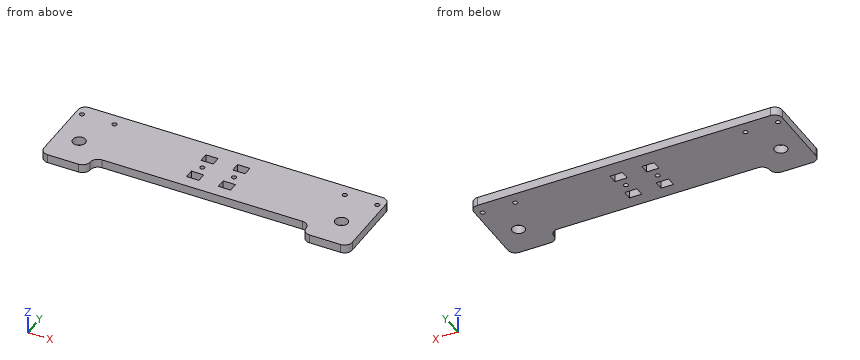
```python
from build123d import *

# Parameters (mm, degrees)
F0_W     = 200
F0_H     = 52
F0_R     = 4.1
F0_W_2   = 8
F0_H_2   = 6
F0_R_2   = 1.5
F1_DEPTH = 5.588
F2_W     = 140
F2_H     = 10
F3_DEPTH = 25
F4_R     = 4.99999


# Not quite as in the source:
# - a fillet or chamfer is up to 0.001 mm smaller than in the source, because OpenCascade refuses the exact size


with BuildPart() as f1:
    # F0 (on Top) → F1 (new body)
    with BuildSketch(Plane.XY):
        Rectangle(F0_W, F0_H)
        with Locations((-85.1, -5.8)):
            Circle(F0_R, mode=Mode.SUBTRACT)
        with Locations((-10.3, -5)):
            Rectangle(F0_W_2, F0_H_2, mode=Mode.SUBTRACT)
        with Locations((10.3, -5)):
            Rectangle(F0_W_2, F0_H_2, mode=Mode.SUBTRACT)
        with Locations((85.1, -5.8)):
            Circle(F0_R, mode=Mode.SUBTRACT)
        with Locations((-10.3, 4)):
            Circle(F0_R_2, mode=Mode.SUBTRACT)
        with Locations((-95.8, 18.2)):
            Circle(F0_R_2, mode=Mode.SUBTRACT)
        with Locations((-74.7, 18.2)):
            Circle(F0_R_2, mode=Mode.SUBTRACT)
        with Locations((-10.3, 13)):
            Rectangle(F0_W_2, F0_H_2, mode=Mode.SUBTRACT)
        with Locations((10.3, 4)):
            Circle(F0_R_2, mode=Mode.SUBTRACT)
        with Locations((10.3, 13)):
            Rectangle(F0_W_2, F0_H_2, mode=Mode.SUBTRACT)
        with Locations((74.7, 18.2)):
            Circle(F0_R_2, mode=Mode.SUBTRACT)
        with Locations((95.8, 18.2)):
            Circle(F0_R_2, mode=Mode.SUBTRACT)
    extrude(amount=F1_DEPTH)

    # F2 (on face) → F3 (cut)
    with BuildSketch(Plane.XY.offset(5.588)):
        with Locations((0, -21)):
            Rectangle(F2_W, F2_H)
    extrude(amount=-F3_DEPTH, mode=Mode.SUBTRACT)

    # F4 (radius 5 in the source; OpenCascade refuses exactly that, so slightly less here)
    f4_edges = [f1.edges().sort_by_distance(p)[0] for p in [
        (-100, 26, 2.794),
        (-100, -26, 2.794),
        (-70, -26, 2.794),
        (-70, -16, 2.794),
        (70, -16, 2.794),
        (70, -26, 2.794),
        (100, -26, 2.794),
        (100, 26, 2.794),
    ]]
    fillet(f4_edges, radius=F4_R)


solid = f1.part
```
Part model, mm, in its own coordinate system. Coordinates: 2 decimals unless noted, no trailing zeros. Order: outer loops, then holes, each group sorted by start corner. A loop starts at its lowest first (then second) coordinate and runs counter-clockwise, first axis right, second up. Notation, with made-up numbers: (35.5, -36.5) - (54.5, -36.5) arc R32 ccw to (54.5, -7.5) - close; hole circle Ø10 at (24.5, -27). An arc over 180 degrees is marked (long way). Return JSON: item names as keys, results as strings. Group by question number.
Item 1: Cut at B-B (y = 12). List the corners of the cut face in (x, z), plus the area to 3 significant figures.
Item 2: Drill centre lines: probe 1 along X at (y, z) = (14, 0.7); probe 2 along Y at (x, z) = (10.3, 1.3); probe 3 along Y at (x, z) = (-74.7, 3.3). Where is each one in solid material? Low to high. Write a range as from..to.
Item 3: Pin check, flat tip, straight feed: pin 1 (1 mm diameter, centred on x = -16, z = 2.5, fed in from -Y). Stop position of the tip, or through.
Item 4: Cut at D-D (x = -63). List the corners of the cut face in (y, z), plus the area to 3 significant figures.
Item 5: Cut at A-A (x = 85.1). List the corners of the cut face in (y, z).
Item 6: Cut at C-C (z = 4.6). State how many separate pieces and enclosed holes the cut face has, plus the area to 3 significant figures.
Check values:
{
 "1": {"outline": "(-100, 0) - (-14.3, 0) - (-14.3, 5.59) - (-100, 5.59) - close; (-6.3, 0) - (6.3, 0) - (6.3, 5.59) - (-6.3, 5.59) - close; (14.3, 0) - (100, 0) - (100, 5.59) - (14.3, 5.59) - close", "area": "1,030 mm2"},
 "2": {"probe 1": "x = -100..-14.3, -6.3..6.3, 14.3..100", "probe 2": "y = -16..-8, -2..2.5, 5.5..10, 16..26", "probe 3": "y = -25.99..16.7, 19.7..26"},
 "3": {"pin 1": "stops at y = -16"},
 "4": {"outline": "(-16, 0) - (26, 0) - (26, 5.59) - (-16, 5.59) - close", "area": "235 mm2"},
 "5": {"outline": "(-26, 0) - (-9.9, 0) - (-9.9, 5.59) - (-26, 5.59) - close; (-1.7, 0) - (26, 0) - (26, 5.59) - (-1.7, 5.59) - close"},
 "6": {"separate pieces": "1", "enclosed holes": "12", "area": "8,640 mm2"}
}
